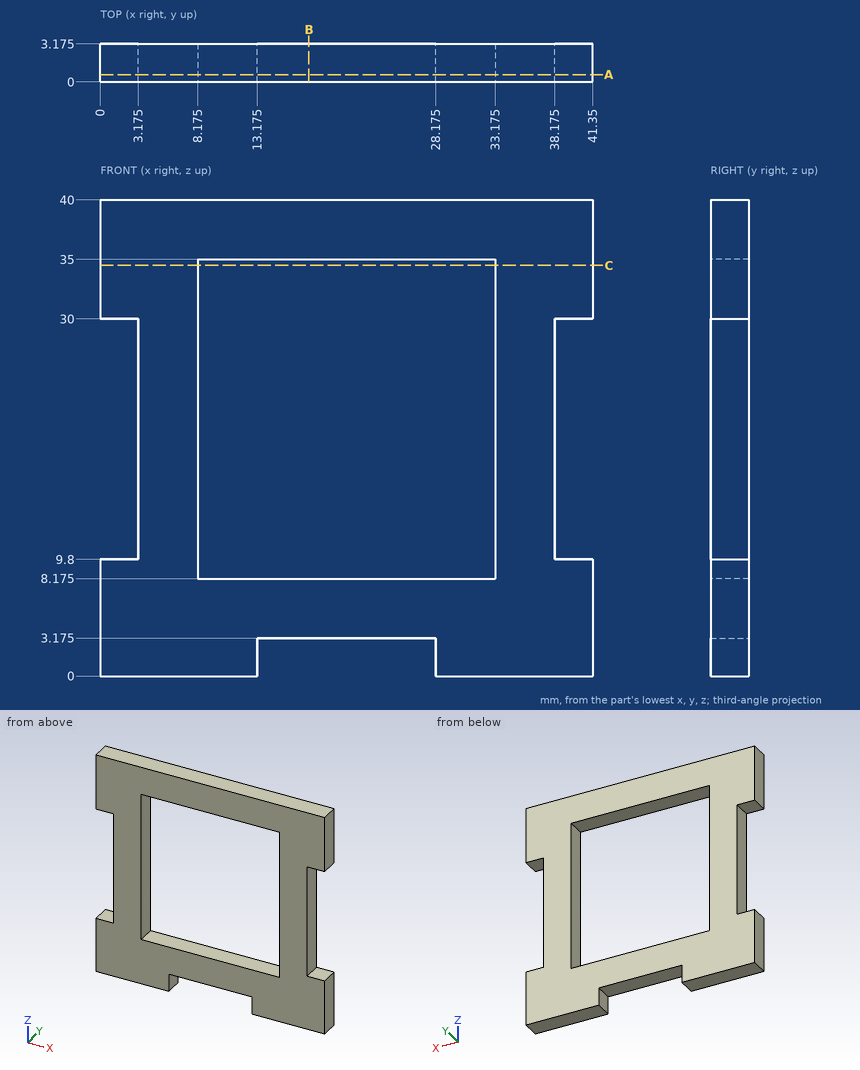
Can you work these out from the drawing? Everything is in mm from the part's minimum corner. Give positions to 0.01 mm unless a question says otherwise; leave off trailing zeros. Order: outer loops, then holes, each group sorted by start corner. A loop starts at its lowest first (then second) coordinate and runs counter-clockwise, first axis right, second up.
1. I need wall thicknesses on L1, parallel to Z at x = 10.5, y = 1.8 (3 decimals); L2, parallel to Z at x = 22, y = 0.75 (3 decimals); L3, parallel to X at y = 1.1, z = 18.5 (3 decimals). Which ranges of each line are inside material? Lowest first, please.
2. Will these pins go through, and if not, where does the flat tip stop? P1, Ø1.6, axis at y = 1.5, z = 20.5, coming from the -X side (3 decimals); P2, Ø1, axis at y = 2, z = 23.5, coming from the +X side (3 decimals).
3. Suppose I cut it at B-B (x = 17.5). List the corners of the cut face in (y, z) for me (3 decimals).
4. Suppose I cut it at A-A (y = 0.6). List the corners of the cut face in (x, z) for me (3 decimals).
5. Suppose I cut it at C-C (z = 34.5). List the corners of the cut face in (x, y) for me (3 decimals), plus the area to 3 significant figures.
Solved:
1. L1: z = 0 to 8.175, 35 to 40
1. L2: z = 3.175 to 8.175, 35 to 40
1. L3: x = 3.175 to 8.175, 33.175 to 38.175
2. P1: stops at x = 3.175
2. P2: stops at x = 38.175
3. outline: (0, 3.175) - (3.175, 3.175) - (3.175, 8.175) - (0, 8.175) - close; (0, 35) - (3.175, 35) - (3.175, 40) - (0, 40) - close
4. outline: (0, 0) - (13.175, 0) - (13.175, 3.175) - (28.175, 3.175) - (28.175, 0) - (41.35, 0) - (41.35, 9.8) - (38.175, 9.8) - (38.175, 30) - (41.35, 30) - (41.35, 40) - (0, 40) - (0, 30) - (3.175, 30) - (3.175, 9.8) - (0, 9.8) - close; hole (8.175, 8.175) - (33.175, 8.175) - (33.175, 35) - (8.175, 35) - close
5. outline: (0, 0) - (8.175, 0) - (8.175, 3.175) - (0, 3.175) - close; (33.175, 0) - (41.35, 0) - (41.35, 3.175) - (33.175, 3.175) - close
5. area: 51.9 mm2
